Geometry check sheet. Reference: the model listing, model coordinates, mm. A direction names the side the tool comes from. Give positions to 0.01 mm unless a question says otherwise; leave off trailing zeros. Write each loop counter-clockwise with the first axis right and the second up, starting at its lowest first coordinate (ties: lowest second). Pieces come first, ordered by that corner, then holes. Notation, with made-up numbers: (-37, -4) -> (-29, -4) arc R7 cw to (-29, 1) -> close; hole circle Ø6 at (81.25, 71.25). An arc over 180 degrees is marked (long way). Write item = value, one per line. Start each with the question number.
1. Cross-section at D-D, the plane y = -12. Record the cut outline in (x, z).
2. Cross-section at B-B, the plane y = 0. Record the cut outline in (x, z), plus the area to 3 significant figures.
3. Thickness scan on line 1 along X through (y, z) = (16.5, 4.3); line 2 along X through (y, z) = (0.5, 1.45); line 3 along Y through (x, z) = (55, 1.4). Record the ranges inside material, lowest first.
4. Mould release check, pull along Y, two halves, no side actions. Record for faces 1 (the cylindrical face through (16.475, 17.945, 3.732)), 2 (the flat face through (0, -18, 2.5)): pulls with the +Y half, pulls with the -Y half, needs draft (parallel to the pull), parting line crosses it, or undercut.
5. Cross-section at A-A, the plane x = -80.4. Record the cut outline in (y, z).
6. Set-up check for faces 3 (the flat face through (57, 7, 2.5)), 4 (the cylindrical face through (-17.16, 14.74, 3.73)), 5 (the cylindrical face through (-6.633, -6.083, 2.535)), 6 (the flat face through (-58, 7, 2.5)), 7 (the flat face through (0, 18, 2.5)): record each of +Z, -Z, +X, -X, +Y, -Y from which the full face is reachable in a straight line by a thin tool's end or side.
7. Cross-section at C-C, the plane z = 0.9. Record the cut outline in (x, y).
8. Depth check by flat-ended pin: P1, Ø1.2, axis at x = 33.5, z = 1.5, coming from the -Y side; P2, Ø6.5, axis at x = 9.5, y = 19, coming from the -Z side; P3, Ø6.5, axis at x = -80.4, y = 0, coming from the +Z side; P4, Ø1.5, axis at y = -11, z = 4.5, coming from the -X side. Enter the tip coordinate at first touch or a pass-through.
```python
from build123d import *

# Parameters (mm, degrees)
SKETCH1_W               = 188.4
SKETCH1_H               = 30
BOSS_EXTRUDE1_DEPTH     = 2.5
SKETCH2_R               = 6
SKETCH2_R_2             = 4
CUT_EXTRUDE2_DEPTH      = 96.419547264
SKETCH3_R               = 1.75
BOSS_EXTRUDE4_DEPTH     = 2.5
CUT_EXTRUDE5_DEPTH      = 14.5
CUT_EXTRUDE5_DEPTH_BACK = 14.5
SKETCH5_R               = 9


with BuildPart() as part:
    # Sketch1 → Boss-Extrude1 (new body)
    with BuildSketch(Plane.XY):
        Rectangle(SKETCH1_W, SKETCH1_H)
    extrude(amount=BOSS_EXTRUDE1_DEPTH)

    # Sketch2 → Cut-Extrude2 (cut, through all)
    with BuildSketch(Plane.XY.offset(2.5)):
        with Locations((-55, 0)):
            Circle(SKETCH2_R)
        with Locations(Location((55, 0, 0), (0, 0, 180))):
            Circle(SKETCH2_R)
        Circle(SKETCH2_R)
        with Locations((-80.4, 0)):
            Circle(SKETCH2_R_2)
        with Locations(Location((80.4, 0, 0), (0, 0, 180))):
            Circle(SKETCH2_R_2)
    extrude(amount=-CUT_EXTRUDE2_DEPTH, mode=Mode.SUBTRACT)

    # Sketch3 → Boss-Extrude4 (add)
    with BuildSketch(Plane.XY.offset(2.5)):
        Polygon((-21, 18.5), (-18.5, 21), (18.5, 21), (21, 18.5), (21, -18.5), (18.5, -21), (-18.5, -21), (-21, -18.5), align=None)
        with Locations(Location((16.214466094, 16.214466094, 0), (0, 0, 223.946041773))):
            Circle(SKETCH3_R, mode=Mode.SUBTRACT)
        with Locations(Location((-16.214466094, -16.214466094, 0), (0, 0, 180))):
            Circle(SKETCH3_R, mode=Mode.SUBTRACT)
        with Locations(Location((16.214466094, -16.214466094, 0), (0, 0, 136.053958227))):
            Circle(SKETCH3_R, mode=Mode.SUBTRACT)
        with Locations(Location((-16.214466094, 16.214466094, 0), (0, 0, 180))):
            Circle(SKETCH3_R, mode=Mode.SUBTRACT)
    extrude(amount=BOSS_EXTRUDE4_DEPTH)

    # Sketch5 → Cut-Extrude5 (cut, two sides: drawn at the far end of the back side and taken through both)
    with BuildSketch(Plane(origin=(0, 0, 2.5), x_dir=(-1, 0, 0), z_dir=(0, 0, -1)).offset(-CUT_EXTRUDE5_DEPTH_BACK)):
        with Locations(Location((0, 0, 0), (0, 0, 180))):
            Circle(SKETCH5_R)
    extrude(amount=CUT_EXTRUDE5_DEPTH + CUT_EXTRUDE5_DEPTH_BACK, mode=Mode.SUBTRACT)


solid = part.part
```
Answers:
q1.outline = (-94.2, 0) -> (94.2, 0) -> (94.2, 2.5) -> (21, 2.5) -> (21, 5) -> (-21, 5) -> (-21, 2.5) -> (-94.2, 2.5) -> close
q2.outline = (-94.2, 0) -> (-84.4, 0) -> (-84.4, 2.5) -> (-94.2, 2.5) -> close; (-76.4, 0) -> (-61, 0) -> (-61, 2.5) -> (-76.4, 2.5) -> close; (-49, 0) -> (-9, 0) -> (-9, 5) -> (-21, 5) -> (-21, 2.5) -> (-49, 2.5) -> close; (9, 0) -> (49, 0) -> (49, 2.5) -> (21, 2.5) -> (21, 5) -> (9, 5) -> close; (61, 0) -> (76.4, 0) -> (76.4, 2.5) -> (61, 2.5) -> close; (84.4, 0) -> (94.2, 0) -> (94.2, 2.5) -> (84.4, 2.5) -> close
q2.area = 386 mm^2
q3.line_1 = -21 to -17.94, -14.49 to 14.49, 17.94 to 21
q3.line_2 = -94.2 to -84.37, -76.43 to -60.98, -49.02 to -8.99, 8.99 to 49.02, 60.98 to 76.43, 84.37 to 94.2
q3.line_3 = -15 to -6, 6 to 15
q4.face_1 = undercut
q4.face_2 = needs draft
q5.outline = (-15, 0) -> (-4, 0) -> (-4, 2.5) -> (-15, 2.5) -> close; (4, 0) -> (15, 0) -> (15, 2.5) -> (4, 2.5) -> close
q6.face_3 = +Z, +X, +Y, -Y
q6.face_4 = +Z
q6.face_5 = +Z, -Z
q6.face_6 = +Z, -X, +Y, -Y
q6.face_7 = -Z, +X, -X, +Y
q7.outline = (-94.2, -15) -> (94.2, -15) -> (94.2, 15) -> (-94.2, 15) -> close; hole circle Ø8 at (-80.4, 0); hole circle Ø12 at (-55, 0); hole circle Ø18 at (0, 0); hole circle Ø12 at (55, 0); hole circle Ø8 at (80.4, 0)
q8.P1 = -15
q8.P2 = 2.5
q8.P3 = through
q8.P4 = -21
